The drawing under review shows one solid part. Ordinate dimensions are in mm from its lowest x, y, z. A direction names the side the tool comes from. Coordinates: 2 decimals unless noted, no trailing zeros. Loops run counter-clockwise (first coordinate to the right, second up) from the corner with the lowest first, then second, coordinate; pieces in that order, holes last.
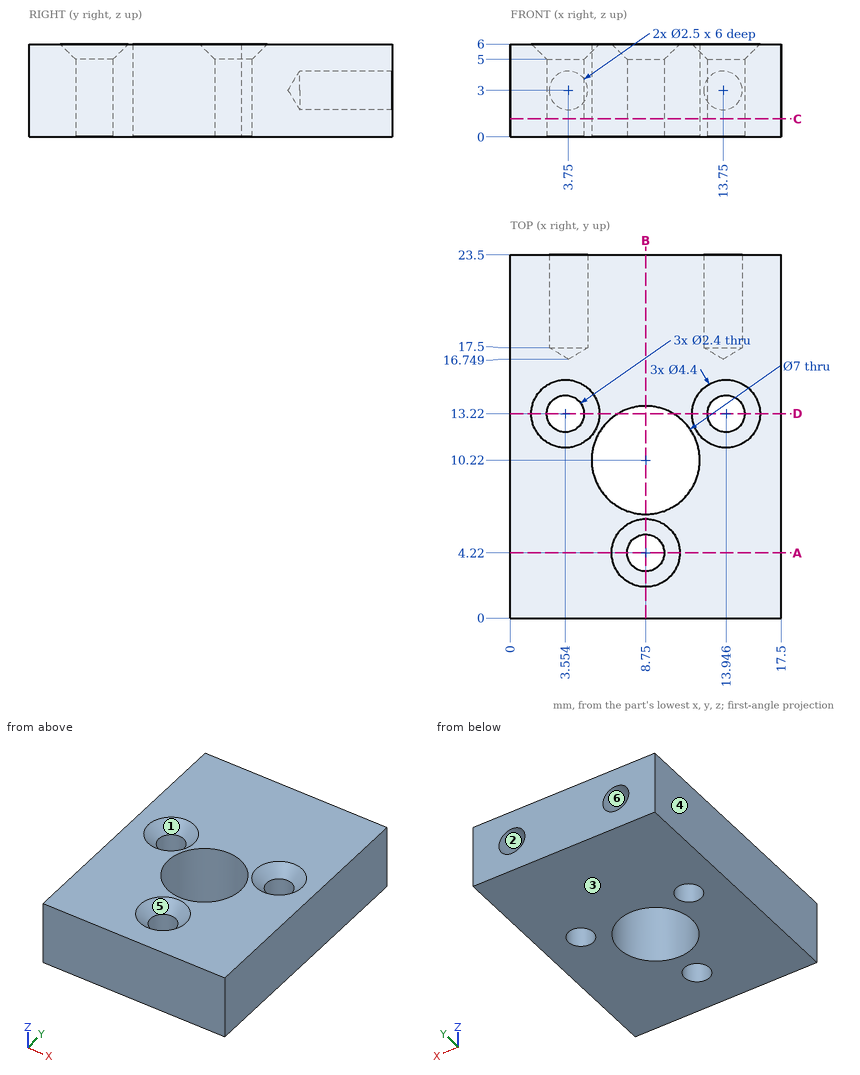
Q1. Clearance check with a flat-ended pin moving along its axis: pin 1 Ø4 at (x, y) = (8.75, 10.22) entering from -Z. State where the tip first meets the part, or that it passes through.
Q2. For line 1 (Y direction, x = 8.75, z = 2.9); line 2 (Y direction, x = 9, z = 5.7); line 3 (X direction, y = 22.25, z = 3.35), list the stretches that pass through material, from the lowest coordinate up.
Q3. Take a section at B-B, the plane x = 8.75. Write out the cut boundary in (y, z).
Q4. The part is to be moulded in two halves that separate along Z. For the marked faces 1, 2, 3 and 4, say which applies: pulls with the +Z half, pulls with the -Z half, needs draft (parallel to the pull), parting line crosses it, or undercut.
Q5. Take a section at A-A, the plane y = 4.22. Write out the cut boundary in (x, z).
Q6. Machinability: for the marked faces 5 and 6, which of the approach directions +Z, -Z, +X, -X, +Y, -Y give a long, thin tool a straight path to every point of the face, cutting with its end or side? Answer none if there is none.
Q7. Take a section at C-C, the plane z = 1.15. Write out the cut boundary in (x, y).
Q8. Take a section at D-D, the plane y = 13.22. Write out the cut boundary in (x, z).
Entries:
1. pin 1: passes through
2. line 1: y = 0 to 3.02, 5.42 to 6.72, 13.72 to 23.5
2. line 2: y = 0 to 2.34, 6.1 to 6.73, 13.71 to 23.5
2. line 3: x = 0 to 2.55, 4.95 to 12.55, 14.95 to 17.5
3. outline: (0, 0) - (3.02, 0) - (3.02, 5) - (2.02, 6) - (0, 6) - close; (5.42, 0) - (6.72, 0) - (6.72, 6) - (6.42, 6) - (5.42, 5) - close; (13.72, 0) - (23.5, 0) - (23.5, 6) - (13.72, 6) - close
4. face 1: pulls with the +Z half
4. face 2: undercut
4. face 3: pulls with the -Z half
4. face 4: needs draft
5. outline: (0, 0) - (7.55, 0) - (7.55, 5) - (6.55, 6) - (0, 6) - close; (9.95, 0) - (17.5, 0) - (17.5, 6) - (10.95, 6) - (9.95, 5) - close
6. face 5: +Z
6. face 6: +Y
7. outline: (0, 0) - (17.5, 0) - (17.5, 23.5) - (0, 23.5) - close; hole circle Ø2.4 at (3.55, 13.22); hole circle Ø7 at (8.75, 10.22); hole circle Ø2.4 at (8.75, 4.22); hole circle Ø2.4 at (13.95, 13.22)
8. outline: (0, 0) - (2.35, 0) - (2.35, 5) - (1.35, 6) - (0, 6) - close; (4.75, 0) - (6.95, 0) - (6.95, 6) - (5.75, 6) - (4.75, 5) - close; (10.55, 0) - (12.75, 0) - (12.75, 5) - (11.75, 6) - (10.55, 6) - close; (15.15, 0) - (17.5, 0) - (17.5, 6) - (16.15, 6) - (15.15, 5) - close
